```python
from build123d import *

# Parameters (mm, degrees)
CROQUIS1_R              = 5
CROQUIS1_R_2            = 7.5
SALIENTE_EXTRUIR1_DEPTH = 10
CROQUIS2_R              = 17.5
CROQUIS2_R_2            = 5
SALIENTE_EXTRUIR2_DEPTH = 30


with BuildPart() as part:
    # Croquis1 → Saliente-Extruir1 (new body)
    with BuildSketch(Plane.XY):
        with BuildLine():
            Line((-212, 17.5), (212, 17.5))
            ThreePointArc((212, 17.5), (229.5, 0), (212, -17.5))
            Line((212, -17.5), (-212, -17.5))
            ThreePointArc((-212, -17.5), (-229.5, 0), (-212, 17.5))
        make_face()
        with Locations((-212, 0)):
            Circle(CROQUIS1_R, mode=Mode.SUBTRACT)
        with Locations((212, 0)):
            Circle(CROQUIS1_R, mode=Mode.SUBTRACT)
        Circle(CROQUIS1_R_2, mode=Mode.SUBTRACT)
    extrude(amount=SALIENTE_EXTRUIR1_DEPTH)

    # Croquis2 → Saliente-Extruir2 (add)
    with BuildSketch(Plane.XY.offset(10)):
        with Locations((-212, 0)):
            Circle(CROQUIS2_R)
        with Locations((-212, 0)):
            Circle(CROQUIS2_R_2, mode=Mode.SUBTRACT)
    extrude(amount=SALIENTE_EXTRUIR2_DEPTH)


solid = part.part
```
The model under review builds one solid part; all positions refer to its coordinate system, in mm. Give positions to 0.01 mm unless a question says otherwise; leave off trailing zeros. Order: outer loops, then holes, each group sorted by start corner. A loop starts at its lowest first (then second) coordinate and runs counter-clockwise, first axis right, second up. Notation, with made-up numbers: (27.25, 80.25) - (33.25, 80.25) arc R13 cw to (33.25, 101.25) - close; hole circle Ø1 at (-22, 61). An arc over 180 degrees is marked (long way). Use CSV: the item, a comma, the result in double quotes. Start each with the question number.
Q1. We need section D-D, the plane x = -150. Write out the cut boundary in (y, z), and give its area (3 significant figures).
Q2. Clearance check with flat-ended pins moving along their axes: pin 1 Ø8 at (x, y) = (85.5, 5) entering from +Z; pin 2 Ø6 at (x, y) = (-212, 0) entering from +Z; pin 3 Ø12 at (y, z) = (11.5, 25.5) entering from +X; pin 4 Ø12 at (y, z) = (-9, 29.5) entering from -X. State where each tip first meets the part, or that it passes through.
Q3. We need section A-A, the plane x = 0. Write out the cut boundary in (y, z).
Q4. We need section C-C, the plane z = 5.5. Write out the cut boundary in (x, y).
Q5. To check wall thickness, follow line 1 along Y through (x, z) = (212, 3); line 2 along X through (y, z) = (2, 6.5); line 3 along X through (y, z) = (0.5, 25.5). State the ranges of each line that lie inside material, in increasing order. Write a range as [from, to].
Q6. We need section B-B, the plane y = 0. Write out the cut boundary in (x, z), and give its area (3 significant figures).
Q7. The part is to be moulded in two halves that separate along X. For faces 1 (the cylindrical face through (-7.493, 0.33, 4.93)), 2 (the flat face through (12, 0, 10)), 3 (the cylindrical face through (216.77, 1.5, 4.93)), 4 (the cylindrical face through (229.496, 0.385, 4.93)), say which applies: +X half, -X half, draft (parallel to the pull), parting line (faces both ways), or undercut.
Outcome:
1,outline,"(-17.5, 0) - (17.5, 0) - (17.5, 10) - (-17.5, 10) - close"
1,area,"350 mm^2"
2,pin 1,"stops at z = 10"
2,pin 2,"passes through"
2,pin 3,"stops at x = -195.39"
2,pin 4,"stops at x = -229.24"
3,outline,"(-17.5, 0) - (-7.5, 0) - (-7.5, 10) - (-17.5, 10) - close; (7.5, 0) - (17.5, 0) - (17.5, 10) - (7.5, 10) - close"
4,outline,"(-212, -17.5) - (212, -17.5) arc R17.5 ccw to (212, 17.5) - (-212, 17.5) arc R17.5 ccw to start; hole circle Ø10 at (-212, 0); hole circle Ø15 at (0, 0); hole circle Ø10 at (212, 0)"
5,line 1,"y = [-17.5, -5], [5, 17.5]"
5,line 2,"x = [-229.39, -216.58], [-207.42, -7.23], [7.23, 207.42], [216.58, 229.39]"
5,line 3,"x = [-229.49, -216.97], [-207.03, -194.51]"
6,outline,"(-229.5, 0) - (-217, 0) - (-217, 40) - (-229.5, 40) - close; (-207, 0) - (-7.5, 0) - (-7.5, 10) - (-194.5, 10) - (-194.5, 40) - (-207, 40) - close; (7.5, 0) - (207, 0) - (207, 10) - (7.5, 10) - close; (217, 0) - (229.5, 0) - (229.5, 10) - (217, 10) - close"
6,area,"4,990 mm^2"
7,face 1,"undercut"
7,face 2,"draft"
7,face 3,"undercut"
7,face 4,"+X half"
